```python
from build123d import *

# Parameters (mm, degrees)
CROQUIS1_W              = 150
CROQUIS1_H              = 390
CROQUIS1_R              = 5
SALIENTE_EXTRUIR1_DEPTH = 5
CROQUIS3_W              = 5
CROQUIS3_H              = 10
CROQUIS3_W_2            = 10
CROQUIS3_H_2            = 5
CORTAR_EXTRUIR1_DEPTH   = 10
CROQUIS4_W              = 10
CROQUIS4_H              = 5
CORTAR_EXTRUIR2_DEPTH   = 10
CROQUIS6_R              = 1.1
CORTAR_EXTRUIR7_DEPTH   = 1


with BuildPart() as part:
    # Croquis1 → Saliente-Extruir1 (new body)
    with BuildSketch(Plane.XY):
        Rectangle(CROQUIS1_W, CROQUIS1_H)
        with Locations((-45, 165)):
            Circle(CROQUIS1_R, mode=Mode.SUBTRACT)
        with Locations((45, 165)):
            Circle(CROQUIS1_R, mode=Mode.SUBTRACT)
        with Locations((-45, -165)):
            Circle(CROQUIS1_R, mode=Mode.SUBTRACT)
        with Locations((45, -165)):
            Circle(CROQUIS1_R, mode=Mode.SUBTRACT)
    extrude(amount=SALIENTE_EXTRUIR1_DEPTH)

    # Croquis3 → Cortar-Extruir1 (cut)
    with BuildSketch(Plane(origin=(0, 0, 0), x_dir=(-1, 0, 0), z_dir=(0, 0, -1))):
        with Locations((-72.5, 100)):
            Rectangle(CROQUIS3_W, CROQUIS3_H)
        with Locations((-72.5, 80)):
            Rectangle(CROQUIS3_W, CROQUIS3_H)
        with Locations((-72.5, 60)):
            Rectangle(CROQUIS3_W, CROQUIS3_H)
        with Locations((-72.5, 40)):
            Rectangle(CROQUIS3_W, CROQUIS3_H)
        with Locations((-72.5, 20)):
            Rectangle(CROQUIS3_W, CROQUIS3_H)
        with Locations((-72.5, 0)):
            Rectangle(CROQUIS3_W, CROQUIS3_H)
        with Locations((-72.5, -20)):
            Rectangle(CROQUIS3_W, CROQUIS3_H)
        with Locations((-72.5, -40)):
            Rectangle(CROQUIS3_W, CROQUIS3_H)
        with Locations((-72.5, -60)):
            Rectangle(CROQUIS3_W, CROQUIS3_H)
        with Locations((-72.5, -80)):
            Rectangle(CROQUIS3_W, CROQUIS3_H)
        with Locations((-72.5, -100)):
            Rectangle(CROQUIS3_W, CROQUIS3_H)
        with Locations((72.5, -100)):
            Rectangle(CROQUIS3_W, CROQUIS3_H)
        with Locations((72.5, -80)):
            Rectangle(CROQUIS3_W, CROQUIS3_H)
        with Locations((72.5, -60)):
            Rectangle(CROQUIS3_W, CROQUIS3_H)
        with Locations((72.5, -40)):
            Rectangle(CROQUIS3_W, CROQUIS3_H)
        with Locations((72.5, -20)):
            Rectangle(CROQUIS3_W, CROQUIS3_H)
        with Locations((72.5, 0)):
            Rectangle(CROQUIS3_W, CROQUIS3_H)
        with Locations((72.5, 20)):
            Rectangle(CROQUIS3_W, CROQUIS3_H)
        with Locations((72.5, 40)):
            Rectangle(CROQUIS3_W, CROQUIS3_H)
        with Locations((72.5, 60)):
            Rectangle(CROQUIS3_W, CROQUIS3_H)
        with Locations((72.5, 80)):
            Rectangle(CROQUIS3_W, CROQUIS3_H)
        with Locations((72.5, 100)):
            Rectangle(CROQUIS3_W, CROQUIS3_H)
        with Locations((-40, -122.5)):
            Rectangle(CROQUIS3_W_2, CROQUIS3_H_2)
        with Locations((-60, -122.5)):
            Rectangle(CROQUIS3_W_2, CROQUIS3_H_2)
        with Locations((-20, -122.5)):
            Rectangle(CROQUIS3_W_2, CROQUIS3_H_2)
        with Locations((0, -122.5)):
            Rectangle(CROQUIS3_W_2, CROQUIS3_H_2)
        with Locations((20, -122.5)):
            Rectangle(CROQUIS3_W_2, CROQUIS3_H_2)
        with Locations((40, -122.5)):
            Rectangle(CROQUIS3_W_2, CROQUIS3_H_2)
        with Locations((60, -122.5)):
            Rectangle(CROQUIS3_W_2, CROQUIS3_H_2)
    extrude(amount=-CORTAR_EXTRUIR1_DEPTH, mode=Mode.SUBTRACT)

    # Croquis4 → Cortar-Extruir2 (cut)
    with BuildSketch(Plane(origin=(0, 0, 0), x_dir=(-1, 0, 0), z_dir=(0, 0, -1))):
        with Locations((-50, 27.5)):
            Rectangle(CROQUIS4_W, CROQUIS4_H)
        with Locations((-30, 27.5)):
            Rectangle(CROQUIS4_W, CROQUIS4_H)
        with Locations((30, 27.5)):
            Rectangle(CROQUIS4_W, CROQUIS4_H)
        with Locations((50, 27.5)):
            Rectangle(CROQUIS4_W, CROQUIS4_H)
    extrude(amount=-CORTAR_EXTRUIR2_DEPTH, mode=Mode.SUBTRACT)

    # Croquis6 → Cortar-Extruir7 (cut)
    with BuildSketch(Plane.XY.offset(5)):
        with Locations((-10.5, -37)):
            Circle(CROQUIS6_R)
        with Locations((10.5, -37)):
            Circle(CROQUIS6_R)
        with Locations((10.5, -49.5)):
            Circle(CROQUIS6_R)
        with Locations((-10.5, -49.5)):
            Circle(CROQUIS6_R)
    extrude(amount=-CORTAR_EXTRUIR7_DEPTH, mode=Mode.SUBTRACT)


solid = part.part
```
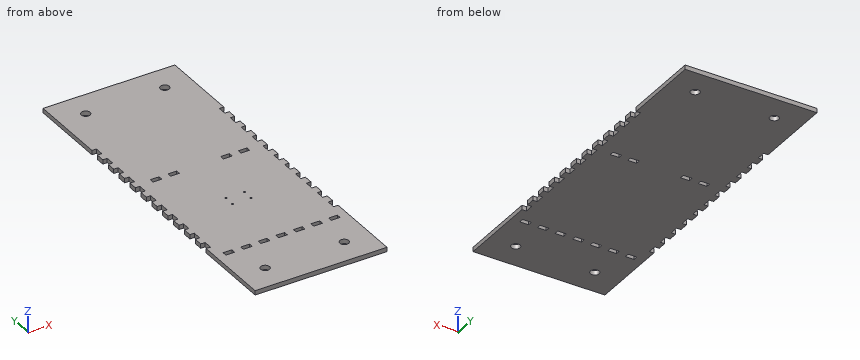
Design review of the part built by this model. Coordinates are the model's own, in mm. Round coordinates to 2 decimals unless told otherwise and drop trailing zeros. Write each loop counter-clockwise with the first axis right and the second up, starting at its lowest first coordinate (ties: lowest second). Pieces come first, ordered by that corner, then holes. Notation, with made-up numbers: (50.25, 27) -> (81.25, 27) arc R24 ccw to (81.25, 44) -> close; hole circle Ø1 at (-11.75, -24). An arc over 180 degrees is marked (long way). Write item = value, one per line. Start each with the question number.
1) Wall thickness on probe 1 along Y at (x, z) = (-10.5, 4.5); probe 2 along Y at (x, z) = (52.5, 1.7); probe 3 along Y at (x, z) = (-4.5, 3.45): over which ranges is each line inside the solid? List them lowest first. Write a range as from..to.
2) Clearance check with flat-ended pins moving along their axes: pin 1 (1.5 mm diameter, centred on y = 2.5, z = 3.5, fed in from -X); pin 2 (2.5 mm diameter, centred on y = -2, z = 2, fed in from +X). State where each tip first meets the part, or that it passes through.
3) Take a section at B-B, the plane z = 2.85. Count the separate pieces of the cut face and the enclosed holes in it, plus the area to 3 significant figures.
4) Take a section at A-A, the plane y = 165. State the section outline as (x, z) points.
Results list:
q1.probe_1 = -195..-50.6, -48.4..-38.1, -35.9..195
q1.probe_2 = -195..25, 30..195
q1.probe_3 = -195..-125, -120..195
q2.pin_1 = -70
q2.pin_2 = 70
q3.separate_pieces = 1
q3.enclosed_holes = 15
q3.area = 56,500 mm²
q4.outline = (-75, 0) -> (-50, 0) -> (-50, 5) -> (-75, 5) -> close; (-40, 0) -> (40, 0) -> (40, 5) -> (-40, 5) -> close; (50, 0) -> (75, 0) -> (75, 5) -> (50, 5) -> close
